Source: CAD feature listing. Evaluate the final solid. Frame: model axes, mm. Give positions to 0.01 mm unless a question says otherwise; leave off trailing zeros. Order: outer loops, then holes, each group sorted by start corner. A loop starts at its lowest first (then second) coordinate and runs counter-clockwise, first axis right, second up. Notation, with made-up numbers: (-31, 89.5) -> (-25, 89.5) arc R14 ccw to (-25, 105.5) -> close; hole circle Ø2 at (-19.75, 1.5). An arc over 180 degrees is marked (long way). Answer in a Markdown table with one row per item.
```python
from build123d import *

# Parameters (mm, degrees)
F0_W     = 114.3
F0_H     = 114.3
F0_W_2   = 103.632
F0_H_2   = 103.632
F1_DEPTH = 27.432
F2_W     = 113.9637678862
F2_H     = 114.4161000848
F3_DEPTH = 2.032
F4_W     = 9.525
F4_H     = 3.2435940627
F4_H_2   = 1.884625411
F4_H_3   = 1.314143768
F4_H_4   = 1.599385288
F4_H_5   = 2.4551072869
F4_H_6   = 2.1698671639
F4_H_7   = 4.1665482581
F4_H_8   = 1.0737287614
F5_DEPTH = 25.4
F6_DEPTH = 25.4


with BuildPart() as f1:
    # F0 (on Top) → F1 (new body)
    with BuildSketch(Plane.XY):
        Rectangle(F0_W, F0_H)
        Rectangle(F0_W_2, F0_H_2, mode=Mode.SUBTRACT)
    extrude(amount=F1_DEPTH)

    # F2 (on Top) → F3 (join)
    with BuildSketch(Plane.XY):
        Rectangle(F2_W, F2_H)
    extrude(amount=F3_DEPTH)

    # F4 (on face) → F5 (join)
    with BuildSketch(Plane.XY.offset(2.032)):
        Polygon((-39.0779674053, 51.816), (-42.291, 51.816), (-42.291, 42.291), (-42.291, 39.0474059373), (-42.291, 29.5224059373), (-42.291, 27.6377805263), (-42.291, 18.1127805263), (-42.291, 16.7986367583), (-42.291, 7.2736367583), (-42.291, 5.6742514703), (-42.291, -3.8507485297), (-42.291, -6.3058558166), (-42.291, -15.8308558166), (-42.291, -18.0007229805), (-42.291, -27.5257229805), (-42.291, -31.6922712386), (-42.291, -41.2172712386), (-42.291, -42.291), (-42.291, -51.816), (-39.0779674053, -51.816), (-39.0779674053, -42.291), (-39.0779674053, -41.2172712386), (-39.0779674053, -31.6922712386), (-39.0779674053, -27.5257229805), (-39.0779674053, -18.0007229805), (-39.0779674053, -15.8308558166), (-39.0779674053, -6.3058558166), (-39.0779674053, -3.8507485297), (-39.0779674053, 5.6742514703), (-39.0779674053, 7.2736367583), (-39.0779674053, 16.7986367583), (-39.0779674053, 18.1127805263), (-39.0779674053, 27.6377805263), (-39.0779674053, 29.5224059373), (-39.0779674053, 39.0474059373), (-39.0779674053, 42.291), align=None)
        with Locations((-47.0535, 40.6692029687)):
            Rectangle(F4_W, F4_H)
        Polygon((-29.5873772812, 42.291), (-39.0779674053, 42.291), (-39.0779674053, 39.0474059373), (-29.5990950418, 39.0474059373), align=None)
        Polygon((-20.097034873, 42.2224297603), (-29.5873772812, 42.291), (-29.5990950418, 39.0474059373), (-20.1204700883, 38.9789203593), align=None)
        with Locations((-47.0535, 28.5800932318)):
            Rectangle(F4_W, F4_H_2)
        Polygon((-20.1204700883, 38.9789203593), (-29.5990950418, 39.0474059373), (-29.6335049177, 29.5224059373), (-20.189288942, 29.4541689733), align=None)
        Polygon((-20.189288942, 29.4541689733), (-29.6335049177, 29.5224059373), (-29.640313288, 27.6377805263), (-20.2029055048, 27.5695927533), align=None)
        with Locations((-47.0535, 17.4557086423)):
            Rectangle(F4_W, F4_H_3)
        Polygon((-20.2029055048, 27.5695927533), (-29.640313288, 27.6377805263), (-29.6747231639, 18.1127805263), (-20.2717243585, 18.0448413672), align=None)
        Polygon((-20.2717243585, 18.0448413672), (-29.6747231639, 18.1127805263), (-29.6794706205, 16.7986367583), (-20.2812191477, 16.7307319), align=None)
        with Locations((-47.0535, 6.4739441143)):
            Rectangle(F4_W, F4_H_4)
        Polygon((-20.2812191477, 16.7307319), (-29.6794706205, 16.7986367583), (-29.7138804964, 7.2736367583), (-20.3500380015, 7.205980514), align=None)
        Polygon((-20.3500380015, 7.205980514), (-29.7138804964, 7.2736367583), (-29.7196584123, 5.6742514703), (-20.3615936825, 5.6066369719), align=None)
        with Locations((-47.0535, -5.0783021731)):
            Rectangle(F4_W, F4_H_5)
        Polygon((-20.3615936825, 5.6066369719), (-29.7196584123, 5.6742514703), (-29.7540682883, -3.8507485297), (-20.4304125362, -3.9181144141), align=None)
        Polygon((-20.4304125362, -3.9181144141), (-29.7540682883, -3.8507485297), (-29.762937573, -6.3058558166), (-20.4481508742, -6.3731576198), align=None)
        with Locations((-47.0535, -16.9157893986)):
            Rectangle(F4_W, F4_H_6)
        Polygon((-20.4481508742, -6.3731576198), (-29.762937573, -6.3058558166), (-29.7973474489, -15.8308558166), (-20.5169697279, -15.8979090058), align=None)
        Polygon((-20.5169697279, -15.8979090058), (-29.7973474489, -15.8308558166), (-29.8051862794, -18.0007229805), (-20.5326471842, -18.0677195336), align=None)
        with Locations((-47.0535, -29.6089971095)):
            Rectangle(F4_W, F4_H_7)
        Polygon((-20.5326471842, -18.0677195336), (-29.8051862794, -18.0007229805), (-29.8395961553, -27.5257229805), (-20.6014660379, -27.5924709196), align=None)
        Polygon((-20.6014660379, -27.5924709196), (-29.8395961553, -27.5257229805), (-29.8546481667, -31.6922712386), (-20.6315696678, -31.7589104257), align=None)
        with Locations((-47.0535, -41.7541356193)):
            Rectangle(F4_W, F4_H_8)
        Polygon((-29.8890580426, -41.2172712386), (-39.0779674053, -41.2172712386), (-39.0779674053, -42.291), (-29.8929369795, -42.291), align=None)
        Polygon((-20.6315696678, -31.7589104257), (-29.8546481667, -31.6922712386), (-29.8890580426, -41.2172712386), (-20.7003885216, -41.2836618117), align=None)
        Polygon((-20.7003885216, -41.2836618117), (-29.8890580426, -41.2172712386), (-29.8929369795, -42.291), (-20.708146294, -42.3573625475), align=None)
    extrude(amount=F5_DEPTH)

    # F4 (on face) → F6 (join)
    with BuildSketch(Plane.XY.offset(2.032)):
        Polygon((-39.0779674053, 51.816), (-42.291, 51.816), (-42.291, 42.291), (-42.291, 39.0474059373), (-42.291, 29.5224059373), (-42.291, 27.6377805263), (-42.291, 18.1127805263), (-42.291, 16.7986367583), (-42.291, 7.2736367583), (-42.291, 5.6742514703), (-42.291, -3.8507485297), (-42.291, -6.3058558166), (-42.291, -15.8308558166), (-42.291, -18.0007229805), (-42.291, -27.5257229805), (-42.291, -31.6922712386), (-42.291, -41.2172712386), (-42.291, -42.291), (-42.291, -51.816), (-39.0779674053, -51.816), (-39.0779674053, -42.291), (-39.0779674053, -41.2172712386), (-39.0779674053, -31.6922712386), (-39.0779674053, -27.5257229805), (-39.0779674053, -18.0007229805), (-39.0779674053, -15.8308558166), (-39.0779674053, -6.3058558166), (-39.0779674053, -3.8507485297), (-39.0779674053, 5.6742514703), (-39.0779674053, 7.2736367583), (-39.0779674053, 16.7986367583), (-39.0779674053, 18.1127805263), (-39.0779674053, 27.6377805263), (-39.0779674053, 29.5224059373), (-39.0779674053, 39.0474059373), (-39.0779674053, 42.291), align=None)
        with Locations((-47.0535, 40.6692029687)):
            Rectangle(F4_W, F4_H)
        Polygon((-29.5873772812, 42.291), (-39.0779674053, 42.291), (-39.0779674053, 39.0474059373), (-29.5990950418, 39.0474059373), align=None)
        Polygon((-20.097034873, 42.2224297603), (-29.5873772812, 42.291), (-29.5990950418, 39.0474059373), (-20.1204700883, 38.9789203593), align=None)
        with Locations((-47.0535, 28.5800932318)):
            Rectangle(F4_W, F4_H_2)
        Polygon((-20.1204700883, 38.9789203593), (-29.5990950418, 39.0474059373), (-29.6335049177, 29.5224059373), (-20.189288942, 29.4541689733), align=None)
        Polygon((-20.189288942, 29.4541689733), (-29.6335049177, 29.5224059373), (-29.640313288, 27.6377805263), (-20.2029055048, 27.5695927533), align=None)
        with Locations((-47.0535, 17.4557086423)):
            Rectangle(F4_W, F4_H_3)
        Polygon((-20.2029055048, 27.5695927533), (-29.640313288, 27.6377805263), (-29.6747231639, 18.1127805263), (-20.2717243585, 18.0448413672), align=None)
        Polygon((-20.2717243585, 18.0448413672), (-29.6747231639, 18.1127805263), (-29.6794706205, 16.7986367583), (-20.2812191477, 16.7307319), align=None)
        with Locations((-47.0535, 6.4739441143)):
            Rectangle(F4_W, F4_H_4)
        Polygon((-20.2812191477, 16.7307319), (-29.6794706205, 16.7986367583), (-29.7138804964, 7.2736367583), (-20.3500380015, 7.205980514), align=None)
        Polygon((-20.3500380015, 7.205980514), (-29.7138804964, 7.2736367583), (-29.7196584123, 5.6742514703), (-20.3615936825, 5.6066369719), align=None)
        with Locations((-47.0535, -5.0783021731)):
            Rectangle(F4_W, F4_H_5)
        Polygon((-20.3615936825, 5.6066369719), (-29.7196584123, 5.6742514703), (-29.7540682883, -3.8507485297), (-20.4304125362, -3.9181144141), align=None)
        Polygon((-20.4304125362, -3.9181144141), (-29.7540682883, -3.8507485297), (-29.762937573, -6.3058558166), (-20.4481508742, -6.3731576198), align=None)
        with Locations((-47.0535, -16.9157893986)):
            Rectangle(F4_W, F4_H_6)
        Polygon((-20.4481508742, -6.3731576198), (-29.762937573, -6.3058558166), (-29.7973474489, -15.8308558166), (-20.5169697279, -15.8979090058), align=None)
        Polygon((-20.5169697279, -15.8979090058), (-29.7973474489, -15.8308558166), (-29.8051862794, -18.0007229805), (-20.5326471842, -18.0677195336), align=None)
        with Locations((-47.0535, -29.6089971095)):
            Rectangle(F4_W, F4_H_7)
        Polygon((-20.5326471842, -18.0677195336), (-29.8051862794, -18.0007229805), (-29.8395961553, -27.5257229805), (-20.6014660379, -27.5924709196), align=None)
        Polygon((-20.6014660379, -27.5924709196), (-29.8395961553, -27.5257229805), (-29.8546481667, -31.6922712386), (-20.6315696678, -31.7589104257), align=None)
        with Locations((-47.0535, -41.7541356193)):
            Rectangle(F4_W, F4_H_8)
        Polygon((-29.8890580426, -41.2172712386), (-39.0779674053, -41.2172712386), (-39.0779674053, -42.291), (-29.8929369795, -42.291), align=None)
        Polygon((-20.6315696678, -31.7589104257), (-29.8546481667, -31.6922712386), (-29.8890580426, -41.2172712386), (-20.7003885216, -41.2836618117), align=None)
        Polygon((-20.7003885216, -41.2836618117), (-29.8890580426, -41.2172712386), (-29.8929369795, -42.291), (-20.708146294, -42.3573625475), align=None)
    extrude(amount=F6_DEPTH)


solid = f1.part
```
(1) Section query C-C (z = 19). Give the number of separate pieces and of enclosed holes in the cut face, plus the area to 3 significant figures.
A:
| item | result |
|---|---|
| separate pieces | 1 |
| enclosed holes | 11 |
| area | 3,660 mm^2 |
(2) Pull-direction query (Y, two-part tool) for faces 1 (the flat face through (-47, 27.638, 15)), 2 (the flat face through (-1, -57.15, 14)); classes: +Y half, -Y half, draft (parallel to the pull), parting line (faces both ways), or undercut.
A:
| item | result |
|---|---|
| face 1 | undercut |
| face 2 | -Y half |
(3) Section query D-D (x = -34.5). Return the cut outline in (y, z).
A:
| item | result |
|---|---|
| outline | (-57.21, 0) -> (57.21, 0) -> (57.21, 2.03) -> (57.15, 2.03) -> (57.15, 27.43) -> (51.82, 27.43) -> (51.82, 2.03) -> (42.29, 2.03) -> (42.29, 27.43) -> (39.05, 27.43) -> (39.05, 2.03) -> (-41.22, 2.03) -> (-41.22, 27.43) -> (-42.29, 27.43) -> (-42.29, 2.03) -> (-51.82, 2.03) -> (-51.82, 27.43) -> (-57.15, 27.43) -> (-57.15, 2.03) -> (-57.21, 2.03) -> close |
(4) Ray query, probe 1 along Y at (x, z) = (-22, 15); probe 2 along X at (y, z) = (-25, 9); probe 3 along X at (y, z) = (6, 18). Return the intervals inside material, ascending.
A:
| item | result |
|---|---|
| probe 1 | y = -57.15 to -51.82, -42.35 to 42.24, 51.82 to 57.15 |
| probe 2 | x = -57.15 to -51.82, -42.29 to -39.08, -29.83 to -20.58, 51.82 to 57.15 |
| probe 3 | x = -57.15 to -39.08, -29.72 to -20.36, 51.82 to 57.15 |
(5) First-contact query: pin 1 Ø5 at (x, y) = (23, 44.5) entering from +Z; pin 2 Ø3 at (x, z) = (15.5, 7) entering from +Y; pin 3 Ø7.5 at (x, z) = (-46.5, 13.5) entering from -Y. Flat tips, straight axial feed; report the tip coordinate or a pass-through.
A:
| item | result |
|---|---|
| pin 1 | stops at z = 2.03 |
| pin 2 | stops at y = 57.15 |
| pin 3 | stops at y = -57.15 |
(6) Section query A-A (x = 38.5). Return the cut outline in (y, z), plus the area to 3 significant figures.
A:
| item | result |
|---|---|
| outline | (-57.21, 0) -> (57.21, 0) -> (57.21, 2.03) -> (57.15, 2.03) -> (57.15, 27.43) -> (51.82, 27.43) -> (51.82, 2.03) -> (-51.82, 2.03) -> (-51.82, 27.43) -> (-57.15, 27.43) -> (-57.15, 2.03) -> (-57.21, 2.03) -> close |
| area | 503 mm^2 |
(7) Section query B-B (y = 25.5). Return the cut outline in (x, z).
A:
| item | result |
|---|---|
| outline | (-57.15, 0) -> (57.15, 0) -> (57.15, 27.43) -> (51.82, 27.43) -> (51.82, 2.03) -> (-20.22, 2.03) -> (-20.22, 27.43) -> (-29.65, 27.43) -> (-29.65, 2.03) -> (-39.08, 2.03) -> (-39.08, 27.43) -> (-42.29, 27.43) -> (-42.29, 2.03) -> (-51.82, 2.03) -> (-51.82, 27.43) -> (-57.15, 27.43) -> close |
